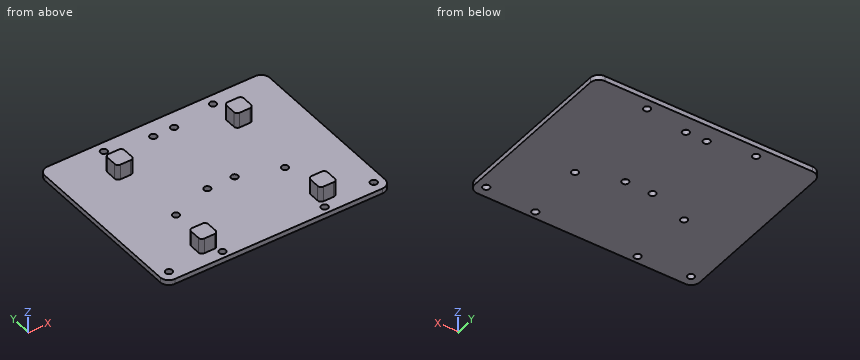
```python
from build123d import *

# Parameters (mm, degrees)
SKETCH1_W           = 66
SKETCH1_H           = 53.2
SKETCH1_R           = 1
SKETCH1_R_2         = 0.98333
SKETCH1_R_3         = 1.011270727
BOSS_EXTRUDE1_DEPTH = 1.5
SKETCH2_W           = 5
SKETCH2_H           = 5
BOSS_EXTRUDE2_DEPTH = 4.5
FILLET1_R           = 1
FILLET2_R           = 2.5


with BuildPart() as part:
    # Sketch1 → Boss-Extrude1 (new body)
    with BuildSketch(Plane.XY.offset(10)):
        with Locations((177.963936399, 293.439054482)):
            Rectangle(SKETCH1_W, SKETCH1_H)
        with Locations((161.947495, 317.06050799)):
            Circle(SKETCH1_R, mode=Mode.SUBTRACT)
        with Locations((193.956452611, 317.06050799)):
            Circle(SKETCH1_R, mode=Mode.SUBTRACT)
        with Locations((174.997800233, 314.982847455)):
            Circle(SKETCH1_R, mode=Mode.SUBTRACT)
        with Locations((181.100928053, 314.982847455)):
            Circle(SKETCH1_R, mode=Mode.SUBTRACT)
        with Locations((173.997800233, 290.965333254)):
            Circle(SKETCH1_R_2, mode=Mode.SUBTRACT)
        with Locations((181.983306885, 290.965333254)):
            Circle(SKETCH1_R, mode=Mode.SUBTRACT)
        with Locations((161.947495, 286.962677261)):
            Circle(SKETCH1_R, mode=Mode.SUBTRACT)
        with Locations((193.956452611, 286.962677261)):
            Circle(SKETCH1_R, mode=Mode.SUBTRACT)
        with Locations((162.947495, 268.970540104)):
            Circle(SKETCH1_R, mode=Mode.SUBTRACT)
        with Locations((192.956452611, 268.970540104)):
            Circle(SKETCH1_R_3, mode=Mode.SUBTRACT)
        with Locations((208.084556857, 269.981810832)):
            Circle(SKETCH1_R, mode=Mode.SUBTRACT)
        with Locations((147.966567684, 269.970540104)):
            Circle(SKETCH1_R, mode=Mode.SUBTRACT)
    extrude(amount=BOSS_EXTRUDE1_DEPTH)

    # Sketch2 → Boss-Extrude2 (add)
    with BuildSketch(Plane.XY.offset(11.5)):
        with Locations((195.50417089, 308.439334712)):
            Rectangle(SKETCH2_W, SKETCH2_H)
        with Locations((160.50417089, 308.439334712)):
            Rectangle(SKETCH2_W, SKETCH2_H)
        with Locations((195.50417089, 273.439334712)):
            Rectangle(SKETCH2_W, SKETCH2_H)
        with Locations((160.50417089, 273.439334712)):
            Rectangle(SKETCH2_W, SKETCH2_H)
    extrude(amount=BOSS_EXTRUDE2_DEPTH)

    # Fillet1
    fillet1_edges = [part.edges().sort_by_distance(p)[0] for p in [
        (163.00417089, 275.939334712, 13.75),
        (158.00417089, 275.939334712, 13.75),
        (158.00417089, 270.939334712, 13.75),
        (163.00417089, 270.939334712, 13.75),
        (158.00417089, 310.939334712, 13.75),
        (158.00417089, 305.939334712, 13.75),
        (163.00417089, 305.939334712, 13.75),
        (163.00417089, 310.939334712, 13.75),
        (198.00417089, 310.939334712, 13.75),
        (193.00417089, 310.939334712, 13.75),
        (193.00417089, 305.939334712, 13.75),
        (198.00417089, 305.939334712, 13.75),
        (198.00417089, 275.939334712, 13.75),
        (193.00417089, 275.939334712, 13.75),
        (193.00417089, 270.939334712, 13.75),
        (198.00417089, 270.939334712, 13.75),
    ]]
    fillet(fillet1_edges, radius=FILLET1_R)

    # Fillet2
    fillet2_edges = [part.edges().sort_by_distance(p)[0] for p in [
        (144.963936399, 320.039054482, 10.75),
        (210.963936399, 320.039054482, 10.75),
        (210.963936399, 266.839054482, 10.75),
        (144.963936399, 266.839054482, 10.75),
    ]]
    fillet(fillet2_edges, radius=FILLET2_R)


solid = part.part
```
The listing builds one solid part. Answer for the finished solid, in the listing's coordinates (mm). Round coordinates to 2 decimals unless told otherwise and drop trailing zeros. Write each loop counter-clockwise with the first axis right and the second up, starting at its lowest first coordinate (ties: lowest second). Pieces come first, ordered by that corner, then holes. Notation, with made-up numbers: (8.25, 10.5) -> (49.25, 10.5) arc R18 cw to (49.25, 18.5) -> close; hole circle Ø3 at (33.25, -10). An arc over 180 degrees is marked (long way). Answer as a JSON object with one key per item and string values. Group by question number.
Q1. Section B-B (y = 309) is taken. Write down the section's boundary in (x, z).
Q2. Section C-C (x = 165) is taken. Write down the section's boundary in (y, z).
Q3. Section A-A (z = 13.05) is taken. Count the separate pieces of the cut face and the enclosed holes in it, plus the area to 3 significant figures.
Q4. Each of these flat-tipped pins is pushed along its axis until it touches: pin 1 Ø0.9 at (x, z) = (195.5, 14) entering from -Y; pin 2 Ø1.8 at (x, y) = (175, 314.98) entering from -Z; pin 3 Ø0.9 at (x, z) = (160, 14) entering from +Y; pin 4 Ø10 at (x, y) = (176.5, 312) entering from +Z. Where does it stop, or does it pass through?
Q5. A straight line is drawn through the part: line 1 along Z through (x, y) = (177, 285). Find the intervals that lie inside material, in ascending order.
Check values:
{
 "1": {"outline": "(144.96, 10) -> (210.96, 10) -> (210.96, 11.5) -> (198, 11.5) -> (198, 16) -> (193, 16) -> (193, 11.5) -> (163, 11.5) -> (163, 16) -> (158, 16) -> (158, 11.5) -> (144.96, 11.5) -> close"},
 "2": {"outline": "(266.84, 10) -> (320.04, 10) -> (320.04, 11.5) -> (266.84, 11.5) -> close"},
 "3": {"separate pieces": "4", "enclosed holes": "0", "area": "96.6 mm^2"},
 "4": {"pin 1": "y = 270.94", "pin 2": "through", "pin 3": "y = 310.94", "pin 4": "z = 11.5"},
 "5": {"line 1": "10 to 11.5"}
}
